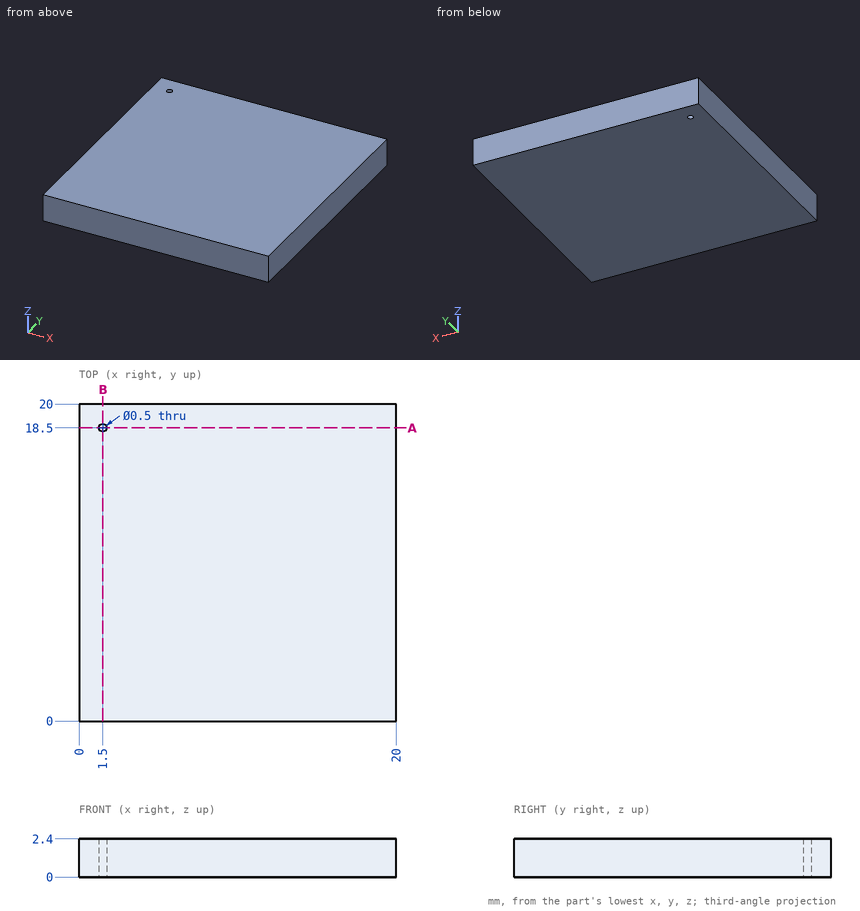
Answer from the drawing. Dimensions are ordinates in mm from the lowest x, y and z of the part. Give positions to 0.01 mm unless a question says otherwise; leave off trailing zeros. Write each loop counter-clockwise with the first axis right and the second up, starting at its lowest first coordinate (ties: lowest second). Pieces come first, ordered by that corner, then holes.
1) Section A-A (y = 18.5) is taken. Write down the section's boundary in (x, z).
2) Find the intervals of material crossed by L1, parallel to Y at x = 1.5, z = 0.8; L2, parallel to X at y = 18.5, z = 0.85, in increasing order.
3) Section B-B (x = 1.5) is taken. Write down the section's boundary in (y, z), and give its area (3 significant figures).
Response:
1. outline: (0, 0) - (1.25, 0) - (1.25, 2.4) - (0, 2.4) - close; (1.75, 0) - (20, 0) - (20, 2.4) - (1.75, 2.4) - close
2. L1: y = 0 to 18.25, 18.75 to 20
2. L2: x = 0 to 1.25, 1.75 to 20
3. outline: (0, 0) - (18.25, 0) - (18.25, 2.4) - (0, 2.4) - close; (18.75, 0) - (20, 0) - (20, 2.4) - (18.75, 2.4) - close
3. area: 46.8 mm2
